```python
from build123d import *

# Parameters (mm, degrees)
F0_W     = 1220
F0_H     = 240
F1_DEPTH = 10
F2_W     = 5
F2_H     = 225
F3_DEPTH = 680
F4_W     = 1195
F4_H     = 225
F4_W_2   = 5
F5_DEPTH = 10
F6_W     = 1190
F6_H     = 680
F7_DEPTH = 5


# Not quite as in the source:
# - a pattern or mirror of a feature is missing from the dataset's text; its kind, count and spacing are read off the source's solid


with BuildPart() as f1:
    # F0 (on Front) → F1 (new body)
    with BuildSketch(Plane.XZ):
        Rectangle(F0_W, F0_H)
    extrude(amount=F1_DEPTH)

    # F2 (on face) → F3 (join)
    with BuildSketch(Plane(origin=(0, 0, 0), x_dir=(-1, 0, 0), z_dir=(0, 1, 0))):
        with Locations((-597.5, -2.5)):
            Rectangle(F2_W, F2_H)
    f3 = extrude(amount=F3_DEPTH)

    # F3_copies: F3 across plane
    add(f3.mirror(Plane(origin=(0, 0, 0), x_dir=(0, 0, -1), z_dir=(-1, 0, 0))))

    # F4 (on face) → F5 (join)
    with BuildSketch(Plane(origin=(0, 680, 0), x_dir=(-1, 0, 0), z_dir=(0, 1, 0))):
        with Locations((2.5, -2.5)):
            Rectangle(F4_W, F4_H)
        with Locations((-597.5, -2.5)):
            Rectangle(F4_W_2, F4_H)
    extrude(amount=F5_DEPTH)

    # F6 (on face) → F7 (join)
    with BuildSketch(Plane(origin=(0, 0, -115), x_dir=(1, 0, 0), z_dir=(0, 0, -1))):
        with Locations((0, -340)):
            Rectangle(F6_W, F6_H)
    extrude(amount=-F7_DEPTH)


solid = f1.part
```
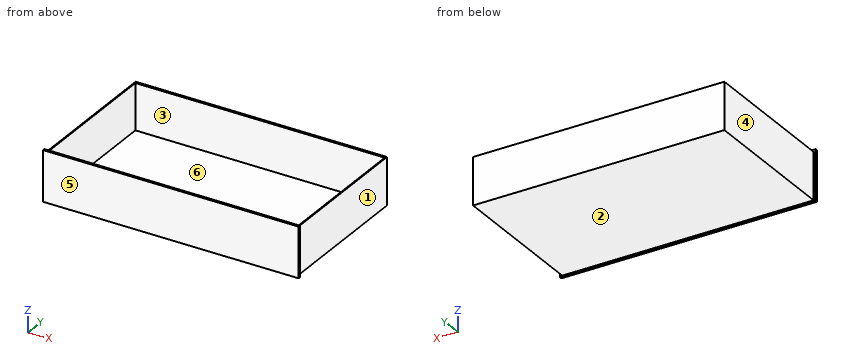
Could you check a few things on this model? Use its own coordinates, in mm. Face numbers are marked on the shaded views. A direction names the side the tool comes from. Give positions to 0.01 mm unless a question says otherwise; leave off trailing zeros. Loops run counter-clockwise (first coordinate to the right, second up) from the corner with the lowest first, then second, coordinate; pieces in that order, holes last. Notation, with made-up numbers: (-2.75, 45.5) - (11.25, 45.5) arc R10 cw to (11.25, 56.5) - close; hole circle Ø6 at (78, 46.5). An arc over 180 degrees is marked (long way). Answer in a Markdown table with one row per item. Add a question column.
Q1. Please list where these lines run through material, in increasing order: L1, parallel to Y at x = 299, z = -56.5; L2, parallel to X at y = 55.5, z = 43.5; L3, parallel to Z at x = -381.5, y = 270.5. Write a range as from..to.
Q2. Which directions (+Z, -Z, +X, -X, +Y, -Y) give clear straight access to the entire face, cutting with the end or side of a thin tool? Please do the marked faces 1, 2 and 3.
Q3. We'd pull the mould along X, two halves only. Please class the marked faces 4, 5 and 6: +X half, -X half, draft (parallel to the pull), parting line (faces both ways), or undercut.
Q4. If we section it at C-C (y = 526): List the corners of the cut face in (x, z) for me.
Q5. If we section it at A-A (z = 33): List the corners of the cut face in (x, y) for me.
Q6. For pin 1 (12 mm diameter, centred on y = 141, z = -96, fed in from -X); pin 2 (10 mm diameter, centred on y = 596, z = 5, fed in from +X); pin 3 (1 mm diameter, centred on x = 293, y = 499.5, fed in from +Z), each with a flat end and sliding along its axis, tell me the tip position at first contact or that it passes through.
Q7. If we section it at B-B (x = 452): List the corners of the cut face in (y, z) for me.
The answers:
| question | item | result |
|---|---|---|
| 1 | L1 | y = -10..0, 680..690 |
| 1 | L2 | x = -600..-595, 595..600 |
| 1 | L3 | z = -115..-110 |
| 2 | face 1 | +Z, -Z, +X, +Y |
| 2 | face 2 | -Z, +X, -X, +Y |
| 2 | face 3 | +Z |
| 3 | face 4 | -X half |
| 3 | face 5 | draft |
| 3 | face 6 | undercut |
| 4 | outline | (-600, -115) - (600, -115) - (600, 110) - (595, 110) - (595, -110) - (-595, -110) - (-595, 110) - (-600, 110) - close |
| 5 | outline | (-610, -10) - (610, -10) - (610, 0) - (600, 0) - (600, 690) - (-600, 690) - (-600, 0) - (-610, 0) - close; hole (-595, 0) - (595, 0) - (595, 680) - (-595, 680) - close |
| 6 | pin 1 | stops at x = -600 |
| 6 | pin 2 | stops at x = 600 |
| 6 | pin 3 | stops at z = -110 |
| 7 | outline | (-10, -120) - (0, -120) - (0, -115) - (690, -115) - (690, 110) - (680, 110) - (680, -110) - (0, -110) - (0, 120) - (-10, 120) - close |
